Check sheet for the modelled part. Datum: model origin and axes. Units: mm. Face numbers are marked on the shaded views. A direction names the side the tool comes from. Coordinates: 2 decimals unless noted, no trailing zeros. Loops run counter-clockwise (first coordinate to the right, second up) from the corner with the lowest first, then second, coordinate; pieces in that order, holes last. Notation, with made-up numbers: M 75,83 L 131,83 A10 cw 131,88 Z; hole C 86,43 d9. An arc over 180 degrees is marked long. Write each question's results on one line, items separated by ' | '. Start each with the question number.
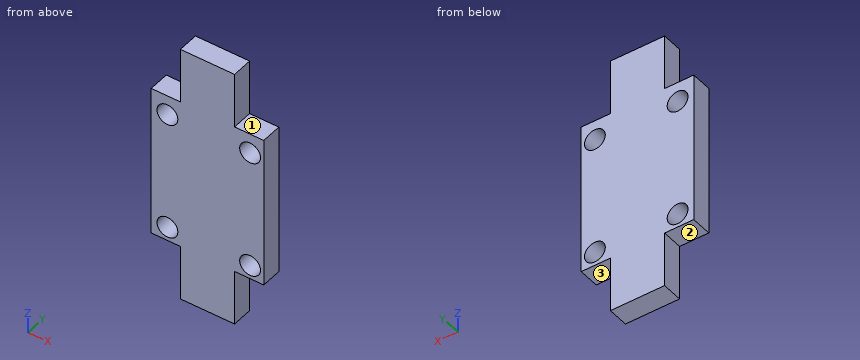
Autodesk Inventor part; units mm, degrees
ref_plane "YZ Plane" through (0, 0, 0) normal (1, 0, 0) x (0, 1, 0)
ref_plane "XZ Plane" through (0, 0, 0) normal (0, 1, 0) x (-1, 0, 0)
ref_plane "XY Plane" through (0, 0, 0) normal (0, 0, 1) x (1, 0, 0)
sketch "Эскиз1" plane through (0, 0, 0) normal (0, 1, 0) x (-1, 0, 0)
  circle A0 centre (6.2967, 9.3442) radius 1.5
  circle A1 centre (-5.6093, 9.3442) radius 1.5
  circle A2 centre (-5.6093, -7.7911) radius 1.5
  circle A3 centre (6.2967, -7.7911) radius 1.5
  line L0 (4.4235, -9.7991) -> (4.4235, -17.7991)
  line L1 (8.6235, -9.7991) -> (4.4235, -9.7991)
  line L2 (8.6235, 12.2009) -> (8.6235, -9.7991)
  line L3 (4.4235, 12.2009) -> (8.6235, 12.2009)
  line L4 (4.4235, 20.2009) -> (4.4235, 12.2009)
  line L5 (-3.3765, 20.2009) -> (4.4235, 20.2009)
  line L6 (-3.3765, 12.2009) -> (-3.3765, 20.2009)
  line L7 (-7.5765, 12.2009) -> (-3.3765, 12.2009)
  line L8 (-7.5765, -9.7991) -> (-7.5765, 12.2009)
  line L9 (-3.3765, -9.7991) -> (-7.5765, -9.7991)
  line L10 (-3.3765, -17.7991) -> (-3.3765, -9.7991)
  line L11 (4.4235, -17.7991) -> (-3.3765, -17.7991)
  point P0 (0, 0)
  point P1 (-15.7765, 1.2009)
extrude "Выдавливание1" add sketch "Эскиз1" along normal blind 3
properties part number "КВ33.044.503 - Прижим ремня" material "Пластик АБС"
1) Gauge pin test, flat ends, axial feed: P1, Ø0.9, axis at x = -7.5, y = 1.5, coming from the -Z side; P2, Ø1.8, axis at x = -6.3, z = -7.79, coming from the +Y side; P3, Ø0.9, axis at x = -6.5, y = 1, coming from the +Z side; P4, Ø1.5, axis at y = 1, z = -15.5, coming from the +X side. Record the tip position at first contact, or that the pin passes through.
2) Section check B-B (z = -8.5). Enter the section's corners in (x, y).
3) Section check A-A (x = 6). Enter the section's corners in (y, z), then the cut area to 3 significant figures.
4) Section check C-C (y = 1.45). Enter the section's corners in (x, z), then the cut area to 3 significant figures.
5) Thickness scan on probe 1 along Z at (x, y) = (5.5, 1.4); probe 2 along Z at (x, y) = (-7, 2.9); probe 3 along X at (y, z) = (0.65, 8.5). Record the ranges inside material, lowest first.
6) Set-up check for the marked faces 1, 2 and 3: record each of +Z, -Z, +X, -X, +Y, -Y from which the full face is reachable in a straight line by a thin tool's end or side.
7) Section check D-D (z = 13). Enter the section's corners in (x, y).
Return value:
1) P1: stops at z = -9.8 | P2: passes through | P3: stops at z = 12.2 | P4: stops at x = 3.38
2) outline: M -8.62,0 L -7.62,0 L -7.62,3 L -8.62,3 Z; M -4.97,0 L 4.29,0 L 4.29,3 L -4.97,3 Z; M 6.93,0 L 7.58,0 L 7.58,3 L 6.93,3 Z
3) outline: M 0,-9.8 L 3,-9.8 L 3,-9.24 L 0,-9.24 Z; M 0,-6.34 L 3,-6.34 L 3,7.9 L 0,7.9 Z; M 0,10.79 L 3,10.79 L 3,12.2 L 0,12.2 Z | area: 48.6 mm2
4) outline: M -8.62,-9.8 L -4.42,-9.8 L -4.42,-17.8 L 3.38,-17.8 L 3.38,-9.8 L 7.58,-9.8 L 7.58,12.2 L 3.38,12.2 L 3.38,20.2 L -4.42,20.2 L -4.42,12.2 L -8.62,12.2 Z; hole C -6.3,-7.79 d3; hole C -6.3,9.34 d3; hole C 5.61,-7.79 d3; hole C 5.61,9.34 d3 | area: 453 mm2
5) probe 1: z = -9.8 to -9.29, -6.3 to 7.85, 10.84 to 12.2 | probe 2: z = -9.8 to -9.12, -6.47 to 8.02, 10.67 to 12.2 | probe 3: x = -8.62 to -7.54, -5.06 to 4.37, 6.85 to 7.58
6) face 1: +Z, +X, +Y, -Y | face 2: -Z, -X, +Y, -Y | face 3: -Z, +X, +Y, -Y
7) outline: M -4.42,0 L 3.38,0 L 3.38,3 L -4.42,3 Z
